Geometry: see drawing. Coordinates: mm, zero at the bounding-box minimum. A direction names the side the tool comes from. Round coordinates to 2 decimals unless told otherwise and drop trailing zeros. Write each loop counter-clockwise with the first axis right and the second up, starting at its lowest first coordinate (ties: lowest second). Pieces come first, ordered by that corner, then holes. Notation, with made-up numbers: M -36.75,55.25 L -32.75,55.25 A28 ccw -32.75,80.25 Z; hole C 22,4.5 d10. An arc over 180 degrees is marked long. Use a Markdown table: item, result.
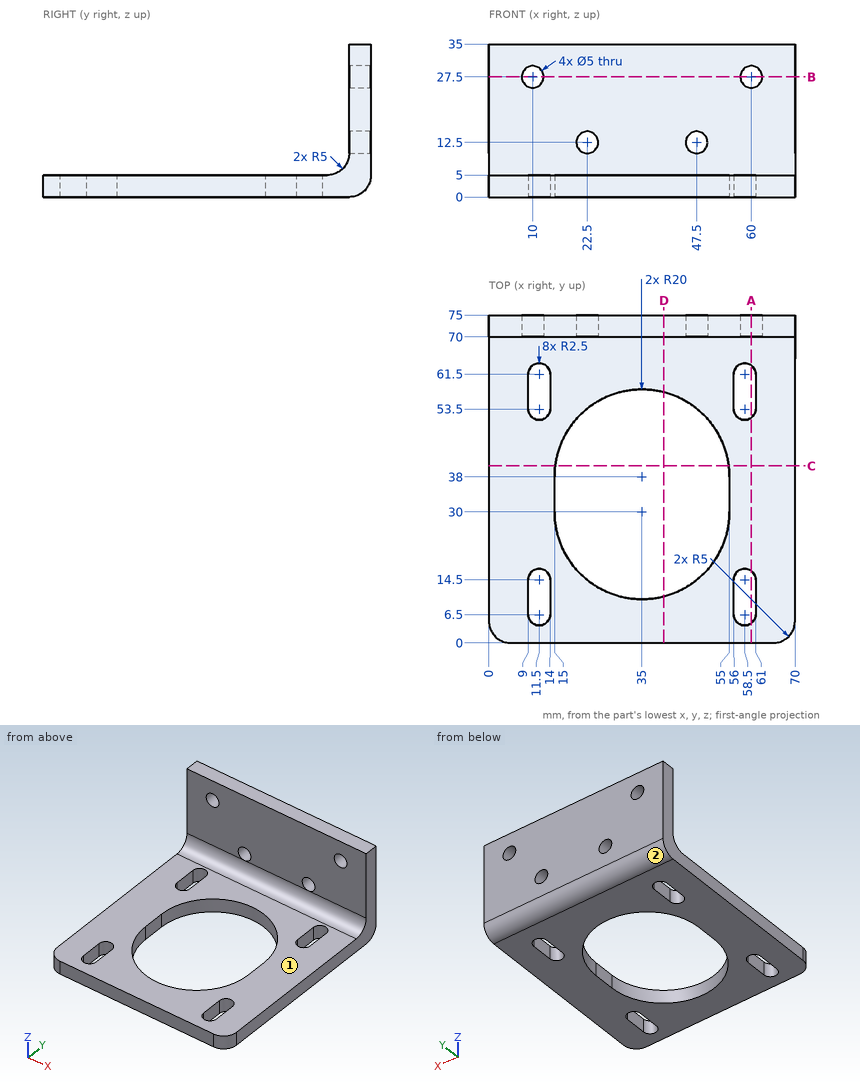
Q1. Section B-B on z = 27.5. Return loops of the section in (x, y), plus the area to 3 significant figures.
Results are:
| item | result |
|---|---|
| outline | M 0,70 L 7.5,70 L 7.5,75 L 0,75 Z; M 12.5,70 L 57.5,70 L 57.5,75 L 12.5,75 Z; M 62.5,70 L 70,70 L 70,75 L 62.5,75 Z |
| area | 300 mm^2 |
Q2. Section D-D on x = 40. Return loops of the section in (y, z), plus the area to 3 significant figures.
Results are:
| item | result |
|---|---|
| outline | M 0,0 L 10.64,0 L 10.64,5 L 0,5 Z; M 57.36,0 L 70,0 A5 ccw 75,5 L 75,35 L 70,35 L 70,10 A5 cw 65,5 L 57.36,5 Z |
| area | 291 mm^2 |
Q3. Line query: L1, parallel to Y at x = 51, z = 27; L2, parallel to Y at x = 25, z = 3.5; L3, parallel to Z at x = 6.5, y = 38. Output: solid intervals per line, ascending.
Results are:
| item | result |
|---|---|
| L1 | 70 to 75 |
| L2 | 0 to 12.68, 55.32 to 74.77 |
| L3 | 0 to 5 |
Q4. First-contact query: pin 1 Ø1.5 at (y, z) = (58.5, 2) entering from -X; pin 2 Ø4.5 at (x, z) = (10, 27.5) entering from +Y; pin 3 Ø6 at (x, y) = (20.5, 66) entering from +Z; pin 4 Ø6 at (x, z) = (47.5, 12.5) entering from -Y. Flat tips, straight axial feed; report the tip coordinate or a pass-through.
Results are:
| item | result |
|---|---|
| pin 1 | x = 0 |
| pin 2 | through |
| pin 3 | z = 7 |
| pin 4 | y = 69.97 |
Q5. Section A-A on x = 60. Return loops of the section in (y, z).
Results are:
| item | result |
|---|---|
| outline | M 0,0 L 4.5,0 L 4.5,5 L 0,5 Z; M 16.5,0 L 51.5,0 L 51.5,5 L 16.5,5 Z; M 63.5,0 L 70,0 A5 ccw 75,5 L 75,25 L 70,25 L 70,10 A5 cw 65,5 L 63.5,5 Z; M 70,30 L 75,30 L 75,35 L 70,35 Z |
Q6. Section C-C on y = 40.5. Return loops of the section in (x, z).
Results are:
| item | result |
|---|---|
| outline | M 0,0 L 15.16,0 L 15.16,5 L 0,5 Z; M 54.84,0 L 70,0 L 70,5 L 54.84,5 Z |
Q7. Reachability of the marked faces 1 and 2 from +Z, -Z, +X, -X, +Y, -Y: full face, straight path, thin tool, end or side. Return the list, or none.
Results are:
| item | result |
|---|---|
| face 1 | +Z, +X, -X, -Y |
| face 2 | -Z, +X, -X, +Y |
